from build123d import *

# Parameters (mm, degrees)
SKETCH1_R           = 4
BOSS_EXTRUDE1_DEPTH = 10
CHAMFER1_SIZE       = 3
CHAMFER1_SIZE2      = 1.091910703
CUT_EXTRUDE1_DEPTH  = 6
CHAMFER2_SIZE       = 1.2
FILLET1_R           = 3
FILLET2_R           = 1.5
BOSS_EXTRUDE2_DEPTH = 1


with BuildPart() as part:
    # Sketch1 → Boss-Extrude1 (new body)
    with BuildSketch(Plane.XY):
        Circle(SKETCH1_R)
    extrude(amount=BOSS_EXTRUDE1_DEPTH)

    # Chamfer1
    chamfer1_edges = [part.edges().sort_by_distance(p)[0] for p in [
        (-4, 0, 10),
    ]]
    chamfer1_side = [part.faces().sort_by_distance(p)[0] for p in [
        (-4, 0, 5),
    ]]
    chamfer(chamfer1_edges, length=CHAMFER1_SIZE, length2=CHAMFER1_SIZE2, reference=chamfer1_side[0])

    # Sketch2 → Cut-Extrude1 (cut)
    with BuildSketch(Plane(origin=(0, 0, 0), x_dir=(-1, 0, 0), z_dir=(0, 0, -1))):
        with BuildLine():
            Line((-1.232882801, -0.55), (1.232882801, -0.55))
            ThreePointArc((1.232882801, -0.55), (0, 1.35), (-1.232882801, -0.55))
        make_face()
    extrude(amount=-CUT_EXTRUDE1_DEPTH, mode=Mode.SUBTRACT)

    # Chamfer2
    chamfer2_edges = [part.edges().sort_by_distance(p)[0] for p in [
        (-4, 0, 0),
    ]]
    chamfer(chamfer2_edges, length=CHAMFER2_SIZE)

    # Fillet1
    fillet1_edges = [part.edges().sort_by_distance(p)[0] for p in [
        (-4, 0, 7),
    ]]
    fillet(fillet1_edges, radius=FILLET1_R)

    # Fillet2
    fillet2_edges = [part.edges().sort_by_distance(p)[0] for p in [
        (-4, 0, 1.2),
    ]]
    fillet(fillet2_edges, radius=FILLET2_R)

    # Sketch3 → Boss-Extrude2 (add)
    with BuildSketch(Plane.XY.offset(10)):
        Polygon((-2.809712327, 0.75), (-0.75, 0.75), (-0.75, 2.809712327), (0.75, 2.809712327), (0.75, 0.75), (2.809712327, 0.75), (2.809712327, -0.75), (0.75, -0.75), (0.75, -2.809712327), (-0.75, -2.809712327), (-0.75, -0.75), (-2.809712327, -0.75), align=None)
    extrude(amount=BOSS_EXTRUDE2_DEPTH)


solid = part.part
The listing builds one solid part. Answer for the finished solid, in the listing's coordinates (mm). A direction names the side the tool comes from. Give positions to 0.01 mm unless a question says otherwise; leave off trailing zeros. Loops run counter-clockwise (first coordinate to the right, second up) from the corner with the lowest first, then second, coordinate; pieces in that order, holes last. Notation, with made-up numbers: (75.5, 1) - (129.5, 1) arc R7 cw to (129.5, 11) - close; hole circle Ø6 at (9.25, -35.5). An arc over 180 degrees is marked (long way). Use one line per item in the form item = value.
1. Find the intervals of material crossed by line 1 along Y through (x, z) = (0, 4.7); line 2 along X through (y, z) = (0, 2); line 3 along Z through (x, y) = (-1.25, -1), in increasing order. Write a range as [from, to].
Calculated:
line_1 = [-4, -0.55], [1.35, 4]
line_2 = [-4, -1.35], [1.35, 4]
line_3 = [0, 10]
2. Which of the six approach directions +Z, -Z, +X, -X, +Y, -Y give full straight-line access (tool end or side, diameter ignored) to faces 5 (the face through (-1.6, 1.6, 10)), 6 (the face through (0.75, 1.8, 10.5)), 7 (the face through (-1.6, -1.5, 10)), 8 (the face through (-2.81, 0, 10.5)), 9 (the face through (0.75, -1.8, 10.5))?
Calculated:
face_5 = +Z, -X, +Y
face_6 = +Z, +X, +Y
face_7 = +Z, -X, -Y
face_8 = +Z, -X, +Y, -Y
face_9 = +Z, +X, -Y
3. Section A-A on z = 3.25 is taken. Give the vertices of the cut face in (x, y), then the cut area to 3 significant figures.
Calculated:
outline = circle Ø8 at (0, 0); hole (-1.23, -0.55) - (1.23, -0.55) arc R1.35 ccw (long way) to start
area = 46.0 mm^2
4. Section B-B on z = 8 is taken. Give the vertices of the cut face in (x, y), then the cut area to 3 significant figures.
Calculated:
outline = circle Ø7.27 at (0, 0)
area = 41.5 mm^2
5. The mould has two halves that part along Y. Classify faces 1 (the face through (1.5, -1.5, 10)), 2 (the face through (1.8, -0.75, 10.5)), 3 (the face through (1.8, 0.75, 10.5)), 4 (the face through (0, 0, 6)): pulls with the +Y half, pulls with the -Y half, needs draft (parallel to the pull), parting line crosses it, or undercut.
Calculated:
face_1 = needs draft
face_2 = pulls with the -Y half
face_3 = pulls with the +Y half
face_4 = undercut
6. Given pin 1 Ø0.8 at (y, z) = (0, 10.5) entering from -X; pin 2 Ø1 at (x, y) = (1.5, -2) entering from +Z; pin 3 Ø0.8 at (x, z) = (-2, 10.5) entering from -Y, each flat-ended and moving along its own axis, determine where each tip first touches the part or whether it passes through.
Calculated:
pin_1 = -2.81
pin_2 = 10
pin_3 = -0.75
